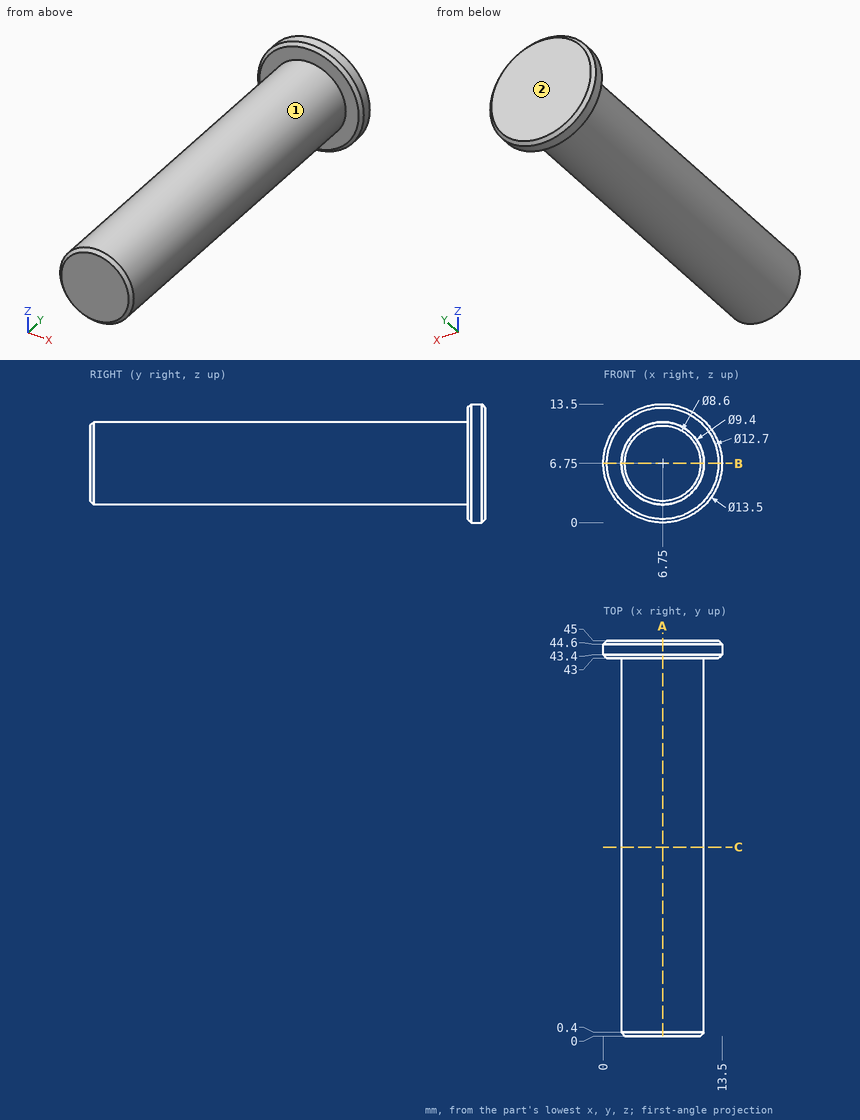
Input: dimensioned drawing with shaded views. Units: mm. Origin: part minimum x, y, z. A direction names the side the tool comes from. Coordinates: 2 decimals unless noted, no trailing zeros. Order: outer loops, then holes, each group sorted by start corner. A loop starts at its lowest first (then second) coordinate and runs counter-clockwise, first axis right, second up.
(1) Section query A-A (x = 6.75). Return the cut outline in (y, z), plus the area to 3 significant figures.
(2) Access query for the marked faces 1 and 2. Directions: +Z, -Z, +X, -X, +Y, -Y. A direction counts if a zero-diameter tool reaches every point of the face in a straight line with its end or side. Return the directions, or none.
(3) First-contact query: pin 1 (2 mm diameter, centred on x = 2, y = 7, fed in from +Z); pin 2 (3 mm diameter, centred on x = 6.5, y = 14.5, fed in from -Z); pin 3 (5 mm diameter, centred on x = 8, y = 21.5, fed in from +Z). Flat tips, straight axial feed; report the tip coordinate or a pass-through.
(4) Section query C-C (y = 21.5). Return the cut outline in (x, z).
(5) Material intervals for probe 1 along Z at (x, y) = (6.75, 41.5); probe 2 along X at (y, z) = (40.5, 6.5); probe 3 along Y at (x, z) = (11.5, 5.25), sorted ascending.
(6) Section query B-B (z = 6.75). Return the cut outline in (x, y).
Solution:
1. outline: (0, 2.45) - (0.4, 2.05) - (43, 2.05) - (43, 0.4) - (43.4, 0) - (44.6, 0) - (45, 0.4) - (45, 13.1) - (44.6, 13.5) - (43.4, 13.5) - (43, 13.1) - (43, 11.45) - (0.4, 11.45) - (0, 11.05) - close
1. area: 431 mm2
2. face 1: -Y
2. face 2: +Z, -Z, +X, -X, +Y
3. pin 1: stops at z = 9.58
3. pin 2: stops at z = 2.05
3. pin 3: stops at z = 11.45
4. outline: circle Ø9.4 at (6.75, 6.75)
5. probe 1: z = 2.05 to 11.45
5. probe 2: x = 2.06 to 11.44
5. probe 3: y = 43 to 45
6. outline: (0, 43.4) - (0.4, 43) - (2.05, 43) - (2.05, 0.4) - (2.45, 0) - (11.05, 0) - (11.45, 0.4) - (11.45, 43) - (13.1, 43) - (13.5, 43.4) - (13.5, 44.6) - (13.1, 45) - (0.4, 45) - (0, 44.6) - close
